Study the drawing (mm; zero at the part's minimum x, y, z) and answer. A direction names the side the tool comes from. Give positions to 0.01 mm unless a question says otherwise; leave off trailing zeros. Write each loop counter-clockwise with the first axis right and the second up, starting at its lowest first coordinate (ties: lowest second). Pieces come first, ordered by that corner, then holes.
1) Given pin 1 Ø2 at (y, z) = (3.5, 9) entering from -X; pin 2 Ø2 at (x, y) = (2.5, 9) entering from +Z; pin 3 Ø2 at (y, z) = (18, 12.5) entering from +X; pin 4 Ø3 at (y, z) = (22, 18) entering from -X, each flat-ended and moving along its own axis, determine where each tip first touches the part or whether it passes through.
2) Find section A-A (x = 3.5). Determine the outline of the cut face in (y, z).
3) Determine the mould class of the marked faces 3, 4 and 5 for opening direction Z: pulls with the +Z half, pulls with the -Z half, needs draft (parallel to the pull), parting line crosses it, or undercut.
4) Straight lines are drawn through the part: probe 1 along Y at (x, z) = (1.45, 9); probe 2 along Z at (x, y) = (0.8, 22) (1 decimal); probe 3 along Z at (x, y) = (2.35, 3.25). For each, find the intervals that lie inside material, in ascending order.
5) Find section B-B (z = 9). Determine the outline of the cut face in (x, y), plus the area to 3 significant figures.
6) Find section C-C (y = 3.5). Determine the outline of the cut face in (x, z).
7) A tool of negligible diameter and unlimited length cuts with its end or side. For the marked faces 1 and 2, from which of +Z, -Z, +X, -X, +Y, -Y can it reach the whole face along a straight path? Write none if from no direction.
8) Find section D-D (x = 0.85). Determine the outline of the cut face in (y, z), plus the area to 3 significant figures.
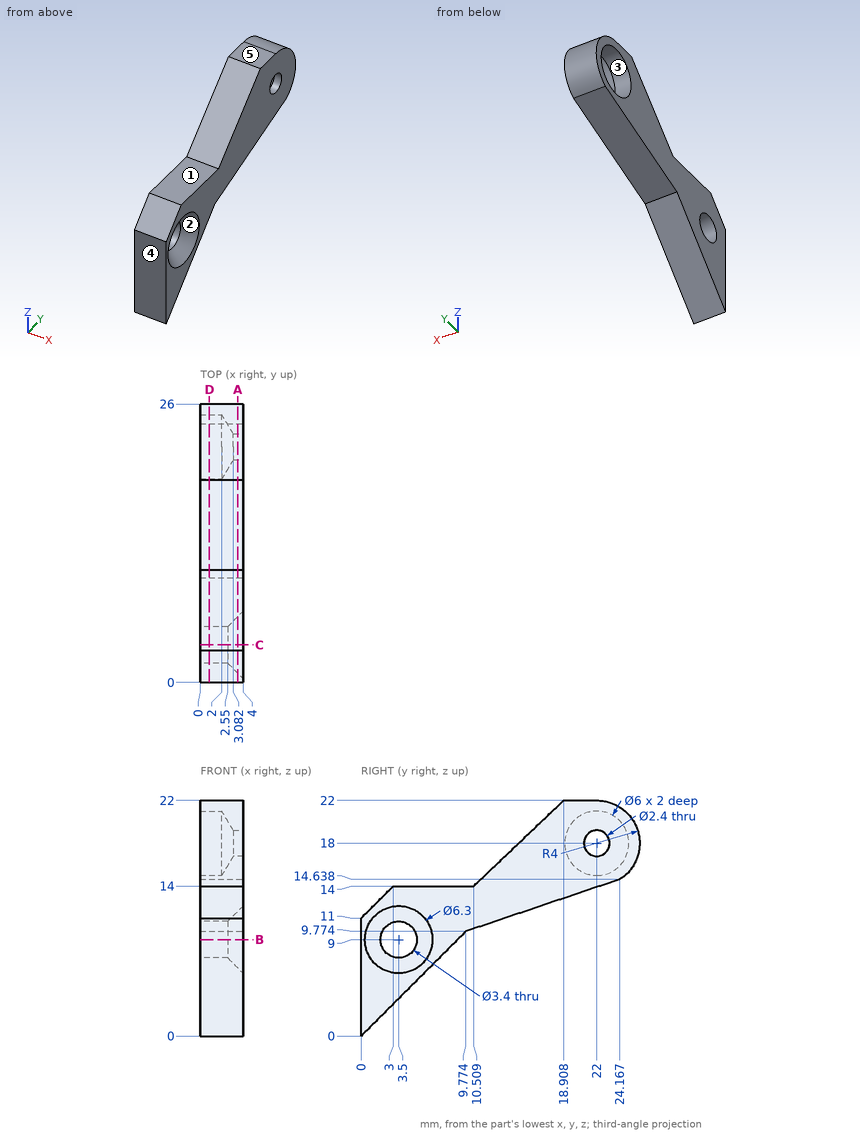
Results:
1. pin 1: passes through
1. pin 2: stops at z = 14
1. pin 3: stops at x = 4
1. pin 4: stops at x = 2.9
2. outline: (0, 0) - (9.77, 9.77) - (24.17, 14.64) arc R4 ccw to (22, 22) - (18.91, 22) - (10.51, 14) - (3, 14) - (0, 11) - close; hole circle Ø5.3 at (3.5, 9); hole circle Ø2.4 at (22, 18)
3. face 3: undercut
3. face 4: needs draft
3. face 5: pulls with the +Z half
4. probe 1: y = 0 to 1.8, 5.2 to 9
4. probe 2: z = 13.9 to 15, 21 to 22
4. probe 3: z = 3.25 to 7.32, 10.68 to 14
5. outline: (0, 0) - (4, 0) - (4, 0.35) - (2.55, 1.8) - (0, 1.8) - close; (0, 5.2) - (2.55, 5.2) - (4, 6.65) - (4, 9) - (0, 9) - close
5. area: 20.3 mm2
6. outline: (0, 3.5) - (4, 3.5) - (4, 5.85) - (2.55, 7.3) - (0, 7.3) - close; (0, 10.7) - (2.55, 10.7) - (4, 12.15) - (4, 14) - (0, 14) - close
7. face 1: +Z, +X, -X, -Y
7. face 2: +X
8. outline: (0, 0) - (9.77, 9.77) - (24.17, 14.64) arc R4 ccw to (22, 22) - (18.91, 22) - (10.51, 14) - (3, 14) - (0, 11) - close; hole circle Ø3.4 at (3.5, 9); hole circle Ø6 at (22, 18)
8. area: 157 mm2
